Could you check a few things on this drawing? It's one solid part, dimensions in mm from its lowest x, y, z. A direction names the side the tool comes from. Give positions to 0.01 mm unless a question says otherwise; leave off trailing zeros. Order: outer loops, then holes, each group sorted by start corner. A loop starts at its lowest first (then second) coordinate and runs counter-clockwise, first axis right, second up.
(1) If I drill on probe 1 along Y at (x, z) = (21, 0.75); probe 2 along Y at (x, z) = (6, 9); probe 3 along Z at (x, y) = (22, 1.75), over which ranges is the centre line in solid material (lowest first)?
(2) Imagine slicing it at D-D, the plane z = 10.5. Write out the boundary of the cut face in (x, y).
(3) Imagine slicing it at A-A, the plane x = 17. Write out the boundary of the cut face in (y, z).
(4) Imagine slicing it at B-B, the plane z = 6. Write out the boundary of the cut face in (x, y).
(5) On a 3-axis mill with a long thin cutter (end or side, diameter ignored), from which of +Z, -Z, +X, -X, +Y, -Y can I reach the whole of each face in a straight line? I mean the marked faces 5 and 6. Say none if no direction works.
(6) If we mould it in two halves opening along Y, with no side actions, what happens to the marked faces 1, 2, 3 and 4? For each: released by +Y, released by -Y, zero draft, split by the parting line, or undercut.
(7) Imagine slicing it at C-C, the plane x = 20.75. Write out the boundary of the cut face in (y, z).
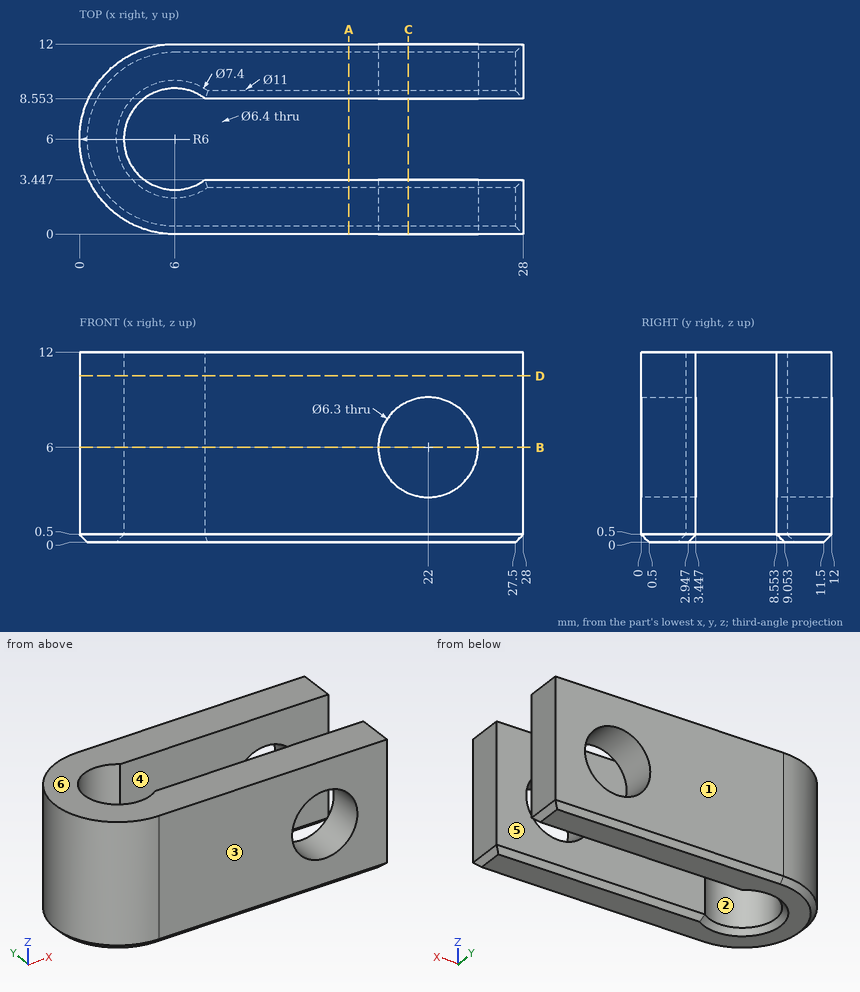
Answer block:
1. probe 1: y = 0 to 3.45, 8.55 to 12
1. probe 2: y = 0 to 2.8, 9.2 to 12
1. probe 3: z = 0 to 2.85, 9.15 to 12
2. outline: (6, 0) - (28, 0) - (28, 3.45) - (7.93, 3.45) arc R3.2 cw (long way) to (7.93, 8.55) - (28, 8.55) - (28, 12) - (6, 12) arc R6 ccw to start
3. outline: (0, 0.5) - (0.5, 0) - (2.95, 0) - (3.45, 0.5) - (3.45, 12) - (0, 12) - close; (8.55, 0.5) - (9.05, 0) - (11.5, 0) - (12, 0.5) - (12, 12) - (8.55, 12) - close
4. outline: (6, 0) - (18.85, 0) - (18.85, 3.45) - (7.93, 3.45) arc R3.2 cw (long way) to (7.93, 8.55) - (18.85, 8.55) - (18.85, 12) - (6, 12) arc R6 ccw to start; (25.15, 0) - (28, 0) - (28, 3.45) - (25.15, 3.45) - close; (25.15, 8.55) - (28, 8.55) - (28, 12) - (25.15, 12) - close
5. face 5: +Z, -Z, +X
5. face 6: +Z, +X, -X, +Y, -Y
6. face 1: released by +Y
6. face 2: undercut
6. face 3: released by -Y
6. face 4: undercut
7. outline: (0, 0.5) - (0.5, 0) - (2.95, 0) - (3.45, 0.5) - (3.45, 3.11) - (0, 3.11) - close; (0, 8.89) - (3.45, 8.89) - (3.45, 12) - (0, 12) - close; (8.55, 0.5) - (9.05, 0) - (11.5, 0) - (12, 0.5) - (12, 3.11) - (8.55, 3.11) - close; (8.55, 8.89) - (12, 8.89) - (12, 12) - (8.55, 12) - close
